The figure shows three views and two pictorial views of one solid part (mm, origin at its lowest corner). Answer the questions. A direction names the side the tool comes from. Coordinates: 2 decimals unless noted, no trailing zeros. Write each loop counter-clockwise with the first axis right and the second up, starting at its lowest first coordinate (ties: lowest second). Pieces come first, ordered by that corner, then holes.
Item 1: Straight lines are drawn through the part: probe 1 along X at (y, z) = (9, 85.5); probe 2 along Z at (x, y) = (24, 10.5); probe 3 along Z at (x, y) = (39.5, 15.5). For each, find the intervals that lie inside material, in ascending order.
Item 2: Determine the mould class of the marked faces 1, 2 and 3 for opening direction X: released by +X, released by -X, zero draft, split by the parting line, or undercut.
Item 3: A tool of negligible diameter and unlimited length cuts with its end or side. For the marked faces 4 and 5, from which of +Z, -Z, +X, -X, +Y, -Y can it reach the whole face along a straight path? Write none if from no direction.
Item 4: Each of these flat-tipped pins is pushed along its axis until it touches: P1, Ø0.6, axis at y = 9.5, z = 2.5, coming from the -X side; P2, Ø10, axis at x = 48.5, y = 6, coming from the -Z side. Where does it stop, or does it pass through?
Item 5: Section B-B (y = 17.75) is taken. Give the vertices of the cut face in (x, z), then the cut area to 3 significant figures.
Item 6: Section C-C (x = 96) is taken. Give the vertices of the cut face in (y, z), then the cut area to 3 significant figures.
Item 7: Section A-A (z = 41.5) is taken. Give the vertices of the cut face in (x, y).
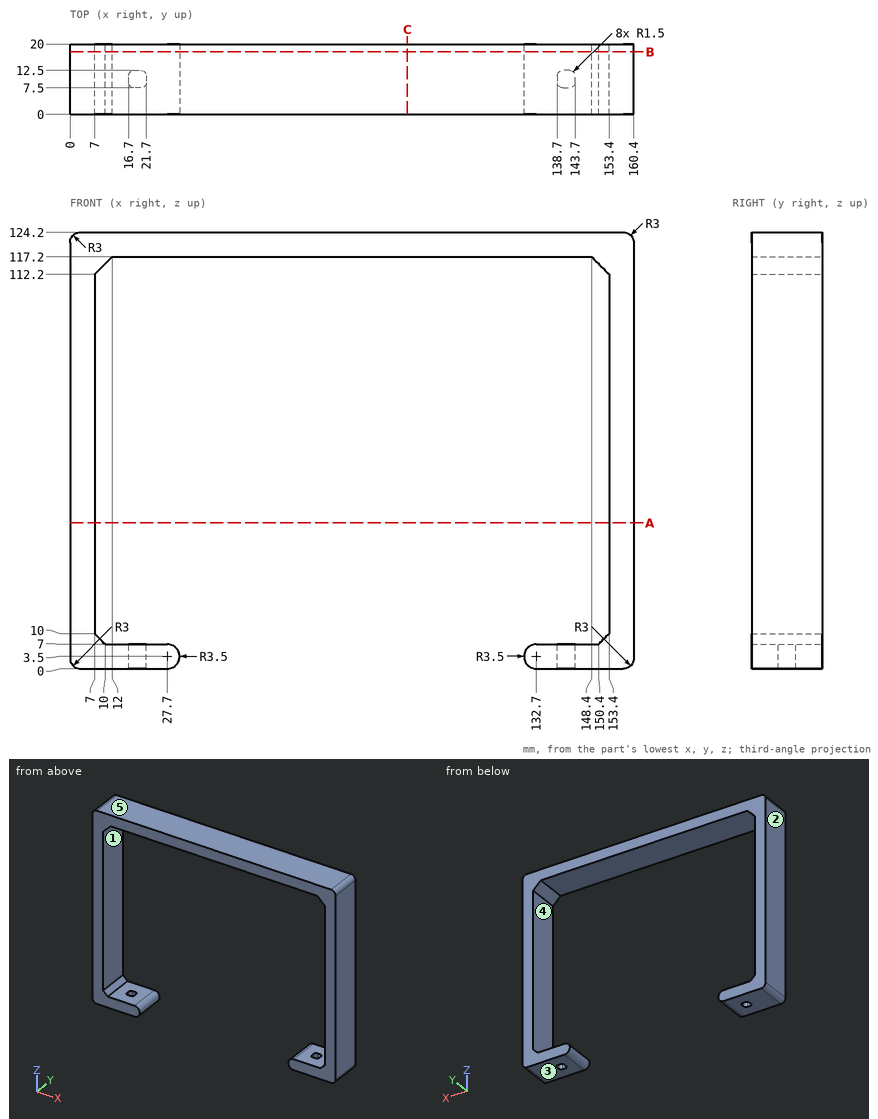
Established:
1. probe 1: x = 0 to 7, 153.4 to 160.4
1. probe 2: z = 0 to 7, 117.2 to 124.2
1. probe 3: z = 117.2 to 124.2
2. face 1: undercut
2. face 2: released by -X
2. face 3: zero draft
3. face 4: +Y, -Y
3. face 5: +Z, +X, -X, +Y, -Y
4. P1: stops at x = 0.01
4. P2: stops at z = 117.2
5. outline: (0, 3) arc R3 ccw to (3, 0) - (27.7, 0) arc R3.5 ccw to (27.7, 7) - (10, 7) - (7, 10) - (7, 112.2) - (12, 117.2) - (148.4, 117.2) - (153.4, 112.2) - (153.4, 10) - (150.4, 7) - (132.7, 7) arc R3.5 ccw to (132.7, 0) - (157.4, 0) arc R3 ccw to (160.4, 3) - (160.4, 121.2) arc R3 ccw to (157.4, 124.2) - (3, 124.2) arc R3 ccw to (0, 121.2) - close
5. area: 3,120 mm2
6. outline: (0, 117.2) - (20, 117.2) - (20, 124.2) - (0, 124.2) - close
6. area: 140 mm2
7. outline: (0, 0) - (7, 0) - (7, 20) - (0, 20) - close; (153.4, 0) - (160.4, 0) - (160.4, 20) - (153.4, 20) - close
